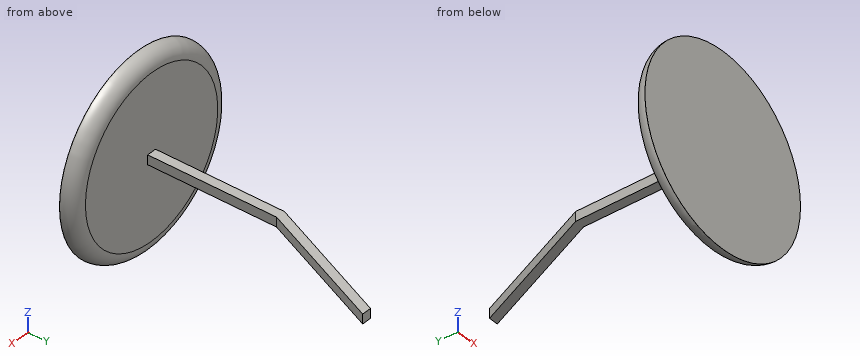
from build123d import *

# Parameters (mm, degrees)
SKETCH_R          = 20
PAD_DEPTH         = 3
PAD001_DEPTH      = 1
PAD001_DEPTH_BACK = 1
FILLET_R          = 2.99


with BuildPart() as part:
    # Sketch → Pad (new body)
    with BuildSketch(Plane.XZ):
        Circle(SKETCH_R)
    extrude(amount=-PAD_DEPTH)

    # Sketch001 → Pad001 (join, two sides)
    with BuildSketch(Plane.XY) as pad001_sk:
        Polygon((-1, 0), (1, 0), (1, 30), (12.736545, 57.608939), (10.736545, 57.608939), (-1, 30), align=None)
    extrude(amount=PAD001_DEPTH)
    extrude(pad001_sk.sketch, amount=-PAD001_DEPTH_BACK)

    # Fillet
    fillet_edges = [part.edges().sort_by_distance(p)[0] for p in [
        (-20, 3, 0),
    ]]
    fillet(fillet_edges, radius=FILLET_R)


solid = part.part
Geometry check sheet. Reference: the model listing, model coordinates, mm. Give positions to 0.01 mm unless a question says otherwise; leave off trailing zeros. Loops run counter-clockwise (first coordinate to the right, second up) from the corner with the lowest first, then second, coordinate; pieces in that order, holes last. Notation, with made-up numbers: (79, 15) -> (135, 15) arc R22 ccw to (135, 21) -> close; hole circle Ø7 at (-31, 80). An arc over 180 degrees is marked (long way). Answer in a Markdown table with one row per item. Add a question column.
1) Cross-section at C-C on y = 32. Record the boundary of the cut face in (x, z), and give its area (3 significant figures).
2) Material ranges on probe 1 along Y at (x, z) = (11.5, -9); probe 2 along Z at (x, y) = (0, 22); probe 3 along Y at (x, z) = (2.5, -17.5), recorded low to high. Write a range as from..to.
3) Gauge pin test, flat ends, axial feed: P1, Ø7, axis at x = 6.5, y = 23.5, coming from the -Z side (3 decimals); P2, Ø7, axis at x = 9, y = 40.5, coming from the +Z side; P3, Ø10, axis at x = 6, z = 14, coming from the +Y side; P4, Ø2, axis at y = 10.5, z = 0, coming from the +X side. Record the tip position at first contact, or that the pin passes through.
Outcome:
| question | item | result |
|---|---|---|
| 1 | outline | (-0.15, -1) -> (1.85, -1) -> (1.85, 1) -> (-0.15, 1) -> close |
| 1 | area | 4.00 mm^2 |
| 2 | probe 1 | y = 0..3 |
| 2 | probe 2 | z = -1..1 |
| 2 | probe 3 | y = 0..2.92 |
| 3 | P1 | passes through |
| 3 | P2 | stops at z = 1 |
| 3 | P3 | stops at y = 3 |
| 3 | P4 | stops at x = 1 |
